Input: part model. Units: mm. Frame: model coordinates. Face numbers are marked on the shaded views. A direction names the side the tool comes from. Give positions to 0.01 mm unless a question says otherwise; leave off trailing zeros. Order: outer loops, then holes, each group sorted by start corner. A loop starts at its lowest first (then second) coordinate and runs counter-clockwise, first axis right, second up. Notation, with made-up numbers: M 78.25,-11 L 114.25,-11 A19 cw 114.25,9 Z; hole C 12,27.25 d4. An arc over 180 degrees is marked long. Use a Markdown table: item, result.
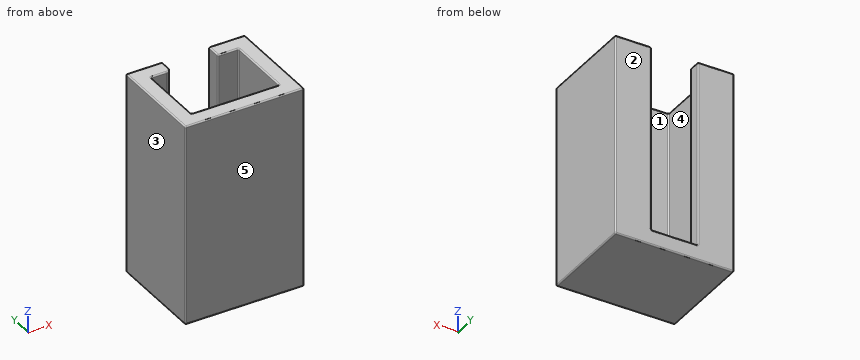
from build123d import *

# Parameters (mm, degrees)
BOSS_EXTRU_1_DEPTH = 36
ESQUISSE2_W        = 23
ESQUISSE2_H        = 19
BOSS_EXTRU_2_DEPTH = 3
CONG_1_R           = 1
CONG_2_R           = 0.25


with BuildPart() as part:
    # Esquisse1 → Boss.-Extru.1 (new body)
    with BuildSketch(Plane.XY):
        Polygon((0, 0), (23, 0), (23, 3), (23, 19), (16, 19), (16, 16), (20, 16), (20, 3), (3, 3), (3, 16), (7, 16), (7, 19), (0, 19), (0, 3), align=None)
    extrude(amount=BOSS_EXTRU_1_DEPTH)

    # Esquisse2 → Boss.-Extru.2 (add)
    with BuildSketch(Plane.XY):
        with Locations((11.5, 9.5)):
            Rectangle(ESQUISSE2_W, ESQUISSE2_H)
    extrude(amount=-BOSS_EXTRU_2_DEPTH)

    # Congé1
    cong_1_edges = [part.edges().sort_by_distance(p)[0] for p in [
        (7, 16, 18),
    ]]
    fillet(cong_1_edges, radius=CONG_1_R)

    # Congé2
    cong_2_edges = [part.edges().sort_by_distance(p)[0] for p in [
        (19.5, 19, 36),
        (16, 17.5, 36),
        (4.5, 16, 0),
        (3, 9.5, 0),
        (11.5, 3, 0),
        (20, 9.5, 0),
        (18, 16, 36),
        (18, 16, 0),
        (16, 17.5, 0),
        (20, 9.5, 36),
        (11.5, 3, 36),
        (23, 0, 16.5),
        (0, 0, 16.5),
        (0, 19, 16.5),
        (7, 19, 18),
        (3, 16, 18),
        (3, 3, 18),
        (20, 3, 18),
        (20, 16, 18),
        (16, 16, 18),
        (16, 19, 18),
        (23, 19, 16.5),
        (3, 9.5, 36),
        (4.5, 16, 36),
        (3.5, 19, 36),
        (0, 9.5, 36),
        (23, 9.5, 36),
        (23, 9.5, -3),
        (11.5, 0, -3),
        (0, 9.5, -3),
        (11.5, 19, -3),
        (11.5, 19, 0),
        (11.5, 0, 36),
        (7, 18, 0),
        (7, 18, 36),
        (6.707106781, 16.292893219, 36),
        (6.707106781, 16.292893219, 0),
    ]]
    fillet(cong_2_edges, radius=CONG_2_R)


solid = part.part
1) Cut plane C-C on z = 28. Return loops of the section in (x, y).
Response values:
| item | result |
|---|---|
| outline | M 0,0.25 A0.25 ccw 0.25,0 L 22.75,0 A0.25 ccw 23,0.25 L 23,18.75 A0.25 ccw 22.75,19 L 16.25,19 A0.25 ccw 16,18.75 L 16,16.25 A0.25 ccw 16.25,16 L 19.75,16 A0.25 cw 20,15.75 L 20,3.25 A0.25 cw 19.75,3 L 3.25,3 A0.25 cw 3,3.25 L 3,15.75 A0.25 cw 3.25,16 L 6,16 A1 ccw 7,17 L 7,18.75 A0.25 ccw 6.75,19 L 0.25,19 A0.25 ccw 0,18.75 Z |
2) Cut plane B-B on x = 18.5. Return loops of the section in (y, z).
Response values:
| item | result |
|---|---|
| outline | M 0,-2.75 A0.25 ccw 0.25,-3 L 18.75,-3 A0.25 ccw 19,-2.75 L 19,35.75 A0.25 ccw 18.75,36 L 16.25,36 A0.25 ccw 16,35.75 L 16,0.25 A0.25 cw 15.75,0 L 3.25,0 A0.25 cw 3,0.25 L 3,35.75 A0.25 ccw 2.75,36 L 0.25,36 A0.25 ccw 0,35.75 Z |
3) Cut plane D-D on x = 10.5. Return loops of the section in (y, z).
Response values:
| item | result |
|---|---|
| outline | M 0,-2.75 A0.25 ccw 0.25,-3 L 18.75,-3 A0.25 ccw 19,-2.75 L 19,-0.25 A0.25 ccw 18.75,0 L 3.25,0 A0.25 cw 3,0.25 L 3,35.75 A0.25 ccw 2.75,36 L 0.25,36 A0.25 ccw 0,35.75 Z |
4) Mould query, pull axis Y, two halves, no side actions, for the marked faces 1, 2 and 3. Classes: released by +Y, released by -Y, zero draft, split by the parting line, or undercut.
Response values:
| item | result |
|---|---|
| face 1 | undercut |
| face 2 | released by +Y |
| face 3 | zero draft |
5) Material intervals for line 1 (X direction, y = 6, z = 29); line 2 (Y direction, x = 18.5, z = 26.5); line 3 (Y direction, x = 14.75, z = 25), sorted ascending. Write a range as from..to.
Response values:
| item | result |
|---|---|
| line 1 | x = 0..3, 20..23 |
| line 2 | y = 0..3, 16..19 |
| line 3 | y = 0..3 |
6) Cut plane A-A on y = 8.75. Return loops of the section in (x, z), and give its area (3 significant figures).
Response values:
| item | result |
|---|---|
| outline | M 0,-2.75 A0.25 ccw 0.25,-3 L 22.75,-3 A0.25 ccw 23,-2.75 L 23,35.75 A0.25 ccw 22.75,36 L 20.25,36 A0.25 ccw 20,35.75 L 20,0.25 A0.25 cw 19.75,0 L 3.25,0 A0.25 cw 3,0.25 L 3,35.75 A0.25 ccw 2.75,36 L 0.25,36 A0.25 ccw 0,35.75 Z |
| area | 285 mm² |
7) First-contact query: pin 1 Ø4.5 at (x, y) = (12.5, 13) entering from +Z; pin 2 Ø5 at (x, z) = (12, 20.5) entering from +Y. Flat tips, straight axial feed; report the tip coordinate or a pass-through.
Response values:
| item | result |
|---|---|
| pin 1 | stops at z = 0 |
| pin 2 | stops at y = 3 |
8) Reachability of the marked faces 4 and 5 from +Z, -Z, +X, -X, +Y, -Y: full face, straight path, thin tool, end or side. Return the list, or none.
Response values:
| item | result |
|---|---|
| face 4 | +Z |
| face 5 | +Z, -Z, +X, -X, -Y |
